Could you check a few things on this model? Use its own coordinates, in mm. Face numbers are marked on the shaded views. Coordinates: 2 decimals unless noted, no trailing zeros. Loops run counter-clockwise (first coordinate to the right, second up) from the corner with the lowest first, then second, coordinate; pieces in that order, holes last.
1) Imagine slicing it at D-D on x = 42.5. Please give me the cut outline in (y, z).
2) Imagine slicing it at A-A on z = -13. Please give me the cut outline in (x, y), plus the area to 3 significant figures.
3) Will these pins go through, and if not, where does the flat tip stop? P1, Ø10, axis at x = 12.5, z = -13.5, coming from the -Y side; P2, Ø1.2, axis at y = 6.5, z = 26.5, coming from the +X side; P3, Ø0.6, axis at y = 4, z = 5, coming from the -X side; P4, Ø3, axis at x = -40, y = 8.5, coming from the -Z side.
4) If I drill on line 1 along Z through (x, y) = (30, 1.5); line 2 along Z through (x, y) = (38.5, 3.25); line 3 along Z through (x, y) = (9.5, 10), over which ranges is the centre line in solid material (lowest first)?
5) Thinking about a two-plate mould opening in Z: for the marked faces 1, 2, 3 and 4, which applies, released by +Z, released by -Z, zero draft, split by the parting line, or undercut?
6) Imagine slicing it at C-C on y = 10. Please give me the cut outline in (x, z).
7) Imagine slicing it at B-B on x = -36.5. Please give me the cut outline in (y, z), plus the area to 3 significant figures.
```python
from build123d import *

# Parameters (mm, degrees)
SKETCH1_W           = 119.2
SKETCH1_H           = 65.04
BOSS_EXTRUDE1_DEPTH = 2
SKETCH2_W           = 59.6
SKETCH2_H           = 2.5
SKETCH2_W_2         = 80
SKETCH2_H_2         = 2
BOSS_EXTRUDE2_DEPTH = 10
FILLET1_R           = 1
SKETCH3_W           = 80
SKETCH3_H           = 2
CUT_EXTRUDE1_DEPTH  = 7
SKETCH4_W           = 80
SKETCH4_H           = 2.5
SKETCH4_W_2         = 8
BOSS_EXTRUDE3_DEPTH = 10
FILLET2_R           = 1
FILLET3_R           = 1
CUT_EXTRUDE2_DEPTH  = 10
CUT_EXTRUDE3_DEPTH  = 10


with BuildPart() as part:
    # Sketch1 → Boss-Extrude1 (new body)
    with BuildSketch(Plane(origin=(0, 0, 0), x_dir=(1, 0, 0), z_dir=(0, 1, 0))):
        Rectangle(SKETCH1_W, SKETCH1_H)
    extrude(amount=BOSS_EXTRUDE1_DEPTH)

    # Sketch2 → Boss-Extrude2 (add)
    with BuildSketch(Plane(origin=(0, 2, 0), x_dir=(1, 0, 0), z_dir=(0, 1, 0))):
        with Locations((0, 28.27)):
            Rectangle(SKETCH2_W, SKETCH2_H)
        with Locations((0, -5.48)):
            Rectangle(SKETCH2_W_2, SKETCH2_H_2)
    extrude(amount=BOSS_EXTRUDE2_DEPTH)

    # Fillet1
    fillet1_edges = [part.edges().sort_by_distance(p)[0] for p in [
        (40, 2, 5.48),
        (0, 2, 4.48),
        (-40, 2, 5.48),
        (-29.8, 2, -28.27),
        (29.8, 2, -28.27),
        (0, 2, -29.52),
    ]]
    fillet(fillet1_edges, radius=FILLET1_R)

    # Sketch3 → Cut-Extrude1 (cut)
    with BuildSketch(Plane(origin=(0, 12, 0), x_dir=(1, 0, 0), z_dir=(0, 1, 0))):
        with Locations((0, -5.48)):
            Rectangle(SKETCH3_W, SKETCH3_H)
        with Locations((0, -9.48)):
            Rectangle(SKETCH3_W, SKETCH3_H)
    extrude(amount=-CUT_EXTRUDE1_DEPTH, mode=Mode.SUBTRACT)

    # Sketch4 → Boss-Extrude3 (add)
    with BuildSketch(Plane(origin=(0, 2, 0), x_dir=(1, 0, 0), z_dir=(0, 1, 0))):
        with Locations((0, -28.77)):
            Rectangle(SKETCH4_W, SKETCH4_H)
        with Locations((52.6, -26.27)):
            Rectangle(SKETCH4_W_2, SKETCH4_H)
    boss_extrude3 = extrude(amount=BOSS_EXTRUDE3_DEPTH)

    # Fillet2
    fillet2_edges = [part.edges().sort_by_distance(p)[0] for p in [
        (-40, 2, 28.77),
        (48.6, 2, 26.27),
        (52.6, 2, 25.02),
        (40, 2, 28.77),
        (0, 2, 27.52),
    ]]
    fillet(fillet2_edges, radius=FILLET2_R)

    # Mirror1: Boss-Extrude3 across plane
    add(boss_extrude3.mirror(Plane.ZY))

    # Fillet3
    fillet3_edges = [part.edges().sort_by_distance(p)[0] for p in [
        (-48.6, 2, 26.27),
        (-52.6, 2, 25.02),
    ]]
    fillet(fillet3_edges, radius=FILLET3_R)

    # Sketch5 → Cut-Extrude2 (cut)
    with BuildSketch(Plane(origin=(0, 2, 0), x_dir=(1, 0, 0), z_dir=(0, 1, 0))):
        with BuildLine():
            Line((46.6, 22.52), (6.311514948, 22.52))
            Line((6.311514948, 22.52), (-46.6, 22.52))
            ThreePointArc((-46.6, 22.52), (-48.721320344, 21.641320344), (-49.6, 19.52))
            Line((-49.6, 19.52), (-49.6, 3.52))
            ThreePointArc((-49.6, 3.52), (-48.721320344, 1.398679656), (-46.6, 0.52))
            Line((-46.6, 0.52), (46.6, 0.52))
            ThreePointArc((46.6, 0.52), (48.721320344, 1.398679656), (49.6, 3.52))
            Line((49.6, 3.52), (49.6, 19.52))
            ThreePointArc((49.6, 19.52), (48.721320344, 21.641320344), (46.6, 22.52))
        make_face()
    extrude(amount=-CUT_EXTRUDE2_DEPTH, mode=Mode.SUBTRACT)

    # Sketch6 → Cut-Extrude3 (cut)
    with BuildSketch(Plane(origin=(0, 2, 0), x_dir=(1, 0, 0), z_dir=(0, 1, 0))):
        with BuildLine():
            Line((54.014213562, -5.94084617), (52.045315698, -3.971948306))
            ThreePointArc((52.045315698, -3.971948306), (51.396469, -3.538402803), (50.631102135, -3.386161868))
            Line((50.631102135, -3.386161868), (46.32782558, -3.386161868))
            ThreePointArc((46.32782558, -3.386161868), (44.913612017, -3.971948306), (44.32782558, -5.386161868))
            Line((44.32782558, -5.386161868), (44.32782558, -20.397912268))
            ThreePointArc((44.32782558, -20.397912268), (44.913612017, -21.812125831), (46.32782558, -22.397912268))
            Line((46.32782558, -22.397912268), (52.6, -22.397912268))
            ThreePointArc((52.6, -22.397912268), (54.014213562, -21.812125831), (54.6, -20.397912268))
            Line((54.6, -20.397912268), (54.6, -7.355059733))
            ThreePointArc((54.6, -7.355059733), (54.447759065, -6.589692868), (54.014213562, -5.94084617))
        make_face()
        with BuildLine():
            Line((39.82782558, -13.44932419), (24.210760832, -13.44932419))
            ThreePointArc((24.210760832, -13.44932419), (23.503654051, -13.742217409), (23.210760832, -14.44932419))
            Line((23.210760832, -14.44932419), (23.210760832, -23.393622011))
            ThreePointArc((23.210760832, -23.393622011), (23.650100661, -24.454282183), (24.710760832, -24.893622011))
            Line((24.710760832, -24.893622011), (39.32782558, -24.893622011))
            ThreePointArc((39.32782558, -24.893622011), (40.388485752, -24.454282183), (40.82782558, -23.393622011))
            Line((40.82782558, -23.393622011), (40.82782558, -14.44932419))
            ThreePointArc((40.82782558, -14.44932419), (40.534932361, -13.742217409), (39.82782558, -13.44932419))
        make_face()
        with BuildLine():
            Line((4.043952302, -24.893622011), (19.660852384, -24.893622011))
            ThreePointArc((19.660852384, -24.893622011), (20.367959165, -24.600728792), (20.660852384, -23.893622011))
            Line((20.660852384, -23.893622011), (20.660852384, -14.321364431))
            ThreePointArc((20.660852384, -14.321364431), (20.221512556, -13.260704259), (19.160852384, -12.821364431))
            Line((19.160852384, -12.821364431), (4.543952302, -12.821364431))
            ThreePointArc((4.543952302, -12.821364431), (3.48329213, -13.260704259), (3.043952302, -14.321364431))
            Line((3.043952302, -14.321364431), (3.043952302, -23.893622011))
            ThreePointArc((3.043952302, -23.893622011), (3.336845521, -24.600728792), (4.043952302, -24.893622011))
        make_face()
        with BuildLine():
            Line((-4.043952302, -24.893622011), (-19.660852384, -24.893622011))
            ThreePointArc((-19.660852384, -24.893622011), (-20.367959165, -24.600728792), (-20.660852384, -23.893622011))
            Line((-20.660852384, -23.893622011), (-20.660852384, -14.321364431))
            ThreePointArc((-20.660852384, -14.321364431), (-20.221512556, -13.260704259), (-19.160852384, -12.821364431))
            Line((-19.160852384, -12.821364431), (-4.543952302, -12.821364431))
            ThreePointArc((-4.543952302, -12.821364431), (-3.48329213, -13.260704259), (-3.043952302, -14.321364431))
            Line((-3.043952302, -14.321364431), (-3.043952302, -23.893622011))
            ThreePointArc((-3.043952302, -23.893622011), (-3.336845521, -24.600728792), (-4.043952302, -24.893622011))
        make_face()
        with BuildLine():
            Line((-39.32782558, -24.893622011), (-24.710760832, -24.893622011))
            ThreePointArc((-24.710760832, -24.893622011), (-23.650100661, -24.454282183), (-23.210760832, -23.393622011))
            Line((-23.210760832, -23.393622011), (-23.210760832, -14.44932419))
            ThreePointArc((-23.210760832, -14.44932419), (-23.503654051, -13.742217409), (-24.210760832, -13.44932419))
            Line((-24.210760832, -13.44932419), (-39.82782558, -13.44932419))
            ThreePointArc((-39.82782558, -13.44932419), (-40.534932361, -13.742217409), (-40.82782558, -14.44932419))
            Line((-40.82782558, -14.44932419), (-40.82782558, -23.393622011))
            ThreePointArc((-40.82782558, -23.393622011), (-40.388485752, -24.454282183), (-39.32782558, -24.893622011))
        make_face()
        with BuildLine():
            Line((-44.32782558, -5.386161868), (-44.32782558, -20.397912268))
            ThreePointArc((-44.32782558, -20.397912268), (-44.913612017, -21.812125831), (-46.32782558, -22.397912268))
            Line((-46.32782558, -22.397912268), (-52.6, -22.397912268))
            ThreePointArc((-52.6, -22.397912268), (-54.014213562, -21.812125831), (-54.6, -20.397912268))
            Line((-54.6, -20.397912268), (-54.6, -7.355059733))
            ThreePointArc((-54.6, -7.355059733), (-54.447759065, -6.589692868), (-54.014213562, -5.94084617))
            Line((-54.014213562, -5.94084617), (-52.045315698, -3.971948306))
            ThreePointArc((-52.045315698, -3.971948306), (-51.396469, -3.538402803), (-50.631102135, -3.386161868))
            Line((-50.631102135, -3.386161868), (-46.32782558, -3.386161868))
            ThreePointArc((-46.32782558, -3.386161868), (-44.913612017, -3.971948306), (-44.32782558, -5.386161868))
        make_face()
    extrude(amount=-CUT_EXTRUDE3_DEPTH, mode=Mode.SUBTRACT)


solid = part.part
```
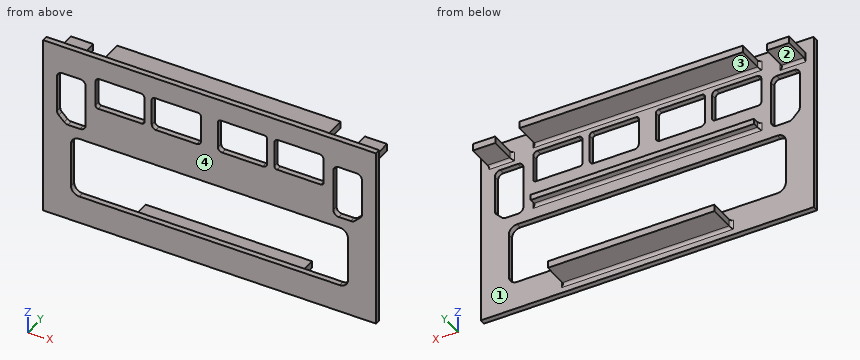
Filled in:
1. outline: (0, -32.52) - (2, -32.52) - (2, -22.52) - (0, -22.52) - close; (0, -0.52) - (2, -0.52) - (2, 32.52) - (0, 32.52) - close
2. outline: (-59.6, 0) - (-49.6, 0) - (-49.6, 2) - (-59.6, 2) - close; (49.6, 0) - (59.6, 0) - (59.6, 2) - (49.6, 2) - close
2. area: 40.0 mm2
3. P1: passes through
3. P2: stops at x = 56.6
3. P3: stops at x = -40
3. P4: stops at z = 27.52
4. line 1: z = -32.52 to -22.52, -0.52 to 13.45, 24.89 to 32.52
4. line 2: z = 4.48 to 6.48, 27.52 to 30.02
4. line 3: z = -29.52 to -27.02, 27.52 to 30.02
5. face 1: undercut
5. face 2: released by -Z
5. face 3: undercut
5. face 4: zero draft
6. outline: (-56.6, 25.02) - (-48.6, 25.02) - (-48.6, 27.52) - (-56.6, 27.52) - close; (-40, 27.52) - (40, 27.52) - (40, 30.02) - (-40, 30.02) - close; (-29.8, -29.52) - (29.8, -29.52) - (29.8, -27.02) - (-29.8, -27.02) - close; (48.6, 25.02) - (56.6, 25.02) - (56.6, 27.52) - (48.6, 27.52) - close
7. outline: (0, -32.52) - (2, -32.52) - (2, -22.52) - (0, -22.52) - close; (0, -0.52) - (2, -0.52) - (2, 3.48) arc R1 cw to (3, 4.48) - (5, 4.48) - (5, 6.48) - (2, 6.48) - (2, 13.45) - (0, 13.45) - close; (0, 24.89) - (2, 24.89) - (2, 26.52) arc R1 cw to (3, 27.52) - (12, 27.52) - (12, 30.02) - (2, 30.02) - (2, 32.52) - (0, 32.52) - close
7. area: 94.6 mm2
